The figure shows three views and two pictorial views of one solid part (mm, origin at its lowest corner). Answer the questions. A direction names the side the tool comes from. Round coordinates to 2 decimals unless told otherwise and drop trailing zeros. Order: outer loops, then holes, each group sorted by start corner. A loop starts at its lowest first (then second) coordinate and runs counter-clockwise, first axis right, second up. Notation, with made-up numbers: (36, -3) -> (54, -3) arc R31 ccw to (54, 28) -> close; hole circle Ø6 at (73, 27). An arc over 180 degrees is marked (long way). One line per item, written item: value. Start each with the question number.
1. Section D-D (z = 17.5) is taken. Give the vertices of the cut face in (x, y), then the cut area to 3 significant figures.
2. Section C-C (x = 14.25) is taken. Give the vertices of the cut face in (y, z), then the cut area to 3 significant figures.
3. Section B-B (y = 1.5) is taken. Give the vertices of the cut face in (x, z), then the cut area to 3 significant figures.
4. The mould has two halves that part along X. Classify the marked faces 4, 5 and 6: released by +X, released by -X, zero draft, split by the parting line, or undercut.
5. Flat-ended cylindrical pins translate along their axes: pin 1 Ø4.5 at (x, z) = (10.5, 10.5) entering from -Y; pin 2 Ø1.5 at (y, z) = (4.5, 8.5) entering from +X; pin 3 Ø3 at (x, z) = (11, 10) entering from +Y. Find the tip coordinate at first contact, or state that the pin passes through.
6. Consider line 1 (Z direction, x = 10.5, y = 5.2); line 2 (Z direction, x = 3.5, y = 4.7). Determine where each line is inside the solid, lowest interval first.
7. For the marked faces 1, 2 and 3, determine the directions among +Z, -Z, +X, -X, +Y, -Y from which every point of the face is accessible in a straight line to the end or side of a thin tool.
8. Section A-A (x = 10.5) is taken. State how many separate pieces and enclosed holes the cut face has, then the cut area to 3 significant figures.
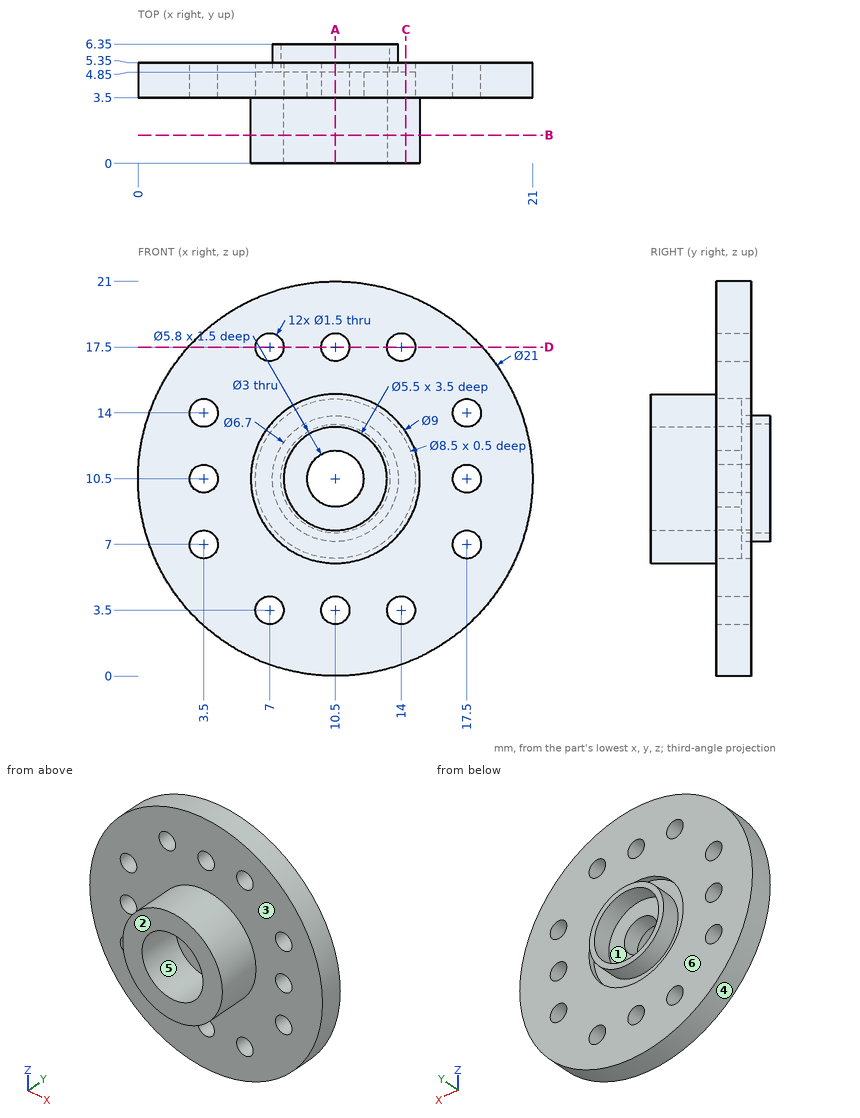
Answer:
1. outline: (2.67, 3.5) -> (6.25, 3.5) -> (6.25, 5.35) -> (2.67, 5.35) -> close; (7.75, 3.5) -> (9.75, 3.5) -> (9.75, 5.35) -> (7.75, 5.35) -> close; (11.25, 3.5) -> (13.25, 3.5) -> (13.25, 5.35) -> (11.25, 5.35) -> close; (14.75, 3.5) -> (18.33, 3.5) -> (18.33, 5.35) -> (14.75, 5.35) -> close
1. area: 20.6 mm^2
2. outline: (0, 8.01) -> (3.5, 8.01) -> (3.5, 4.21) -> (5.35, 4.21) -> (5.35, 8.5) -> (4.85, 8.5) -> (4.85, 12.5) -> (5.35, 12.5) -> (5.35, 16.79) -> (3.5, 16.79) -> (3.5, 12.99) -> (0, 12.99) -> close; (3.5, 0.69) -> (5.35, 0.69) -> (5.35, 2.79) -> (3.5, 2.79) -> close; (3.5, 18.21) -> (5.35, 18.21) -> (5.35, 20.31) -> (3.5, 20.31) -> close
2. area: 46.5 mm^2
3. outline: circle Ø9 at (10.5, 10.5); hole circle Ø5.5 at (10.5, 10.5)
3. area: 39.9 mm^2
4. face 4: split by the parting line
4. face 5: undercut
4. face 6: zero draft
5. pin 1: y = 3.5
5. pin 2: x = 20.93
5. pin 3: y = 4.85
6. line 1: 0 to 2.75, 4.25 to 6.25, 7.15 to 7.6, 13.4 to 13.85, 14.75 to 16.75, 18.25 to 21
6. line 2: 2.67 to 6.25, 7.75 to 9.75, 11.25 to 13.25, 14.75 to 18.33
7. face 1: +Y
7. face 2: +Z, -Z, +X, -X, -Y
7. face 3: -Y
8. separate pieces: 4
8. enclosed holes: 0
8. area: 38.6 mm^2
